Build history of the part. All positions in model axes, mm. Give positions to 0.01 mm unless a question says otherwise; leave off trailing zeros. Order: outer loops, then holes, each group sorted by start corner. A loop starts at its lowest first (then second) coordinate and runs counter-clockwise, first axis right, second up. Notation, with made-up numbers: M 80.5,-37 L 104.5,-37 A21 ccw 104.5,-4 Z; hole C 55,50 d1. An arc over 180 degrees is marked long. One line per item, written item: value.
Solid Edge part; units mm, degrees
sketch "Sketch1" plane through (0, 0, 0) normal (0, 0, 1) x (1, 0, 0)
  circle A0 centre (0, 0) radius 775
  circle A1 centre (0, 0) radius 460
extrude "Protrusion1" add sketch "Sketch1" against normal blind 42
hole "Agujero_1" at (0, 725, 0) direction (0, 0, -1) diameter 30 end up to next
pattern_circular "Pattern1" count 28 over 360 about axis through (0, 0, 0) along (0, 0, -1) of "Agujero_1"
1) Pin check, flat tips, straight feed: pin 1 (4 mm diameter, centred on y = -445.5, z = -35.5, fed in from -X); pin 2 (18 mm diameter, centred on x = -725, y = 0, fed in from -Z); pin 3 (1 mm diameter, centred on y = 342, z = -34.5, fed in from -X); pin 4 (10 mm diameter, centred on x = 324, z = -12.5, fed in from +Y). Stop position of each tip, or through.
Check values:
pin 1: x = -635.56
pin 2: through
pin 3: x = -695.7
pin 4: y = 706.3
2) Saw through at C-C, the plane z = -19.5. Give the number of separate pieces and of enclosed holes in the cut face, then the cut area to 3 significant figures.
Check values:
separate pieces: 1
enclosed holes: 29
area: 1,200,000 mm^2
3) Drill centre lines: probe 1 along Y at (x, z) = (461, -39); probe 2 along X at (y, z) = (-7.5, -11); probe 3 along Y at (x, z) = (-307, -11). Where is each one in solid material? Low to high. Write a range as from..to.
Check values:
probe 1: -622.98..-578.85, -554.81..554.81, 578.85..622.98
probe 2: -774.96..-737.99, -712.01..-459.94, 459.94..712.01, 737.99..774.96
probe 3: -711.6..-666.15, -640.25..-342.57, 342.57..640.25, 666.15..711.6
4) Saw through at A-A, the plane y = -409. Write the cut outline in (x, z), then the cut area to 3 significant figures.
Check values:
outline: M -658.29,-42 L -210.52,-42 L -210.52,0 L -658.29,0 Z; M 210.52,-42 L 658.29,-42 L 658.29,0 L 210.52,0 Z
area: 37,600 mm^2
5) Mould opens along Y. For faces 1 (the face through (-100, -449, -21)), 2 (the face through (-615.01, -471.58, -20.71)), 3 (the face through (334, -334, -42)) say: released by +Y, released by -Y, zero draft, split by the parting line, or undercut.
Check values:
face 1: undercut
face 2: split by the parting line
face 3: zero draft
6) Saw through at B-B, the plane x = -400.5. Write the cut outline in (y, z).
Check values:
outline: M -663.49,-42 L -226.27,-42 L -226.27,0 L -663.49,0 Z; M 226.27,-42 L 663.49,-42 L 663.49,0 L 226.27,0 Z
